Build history of the part. All positions in model axes, mm. Face numbers are marked on the shaded views. Round coordinates to 2 decimals unless told otherwise and drop trailing zeros. Loops run counter-clockwise (first coordinate to the right, second up) from the corner with the lowest first, then second, coordinate; pieces in that order, holes last.
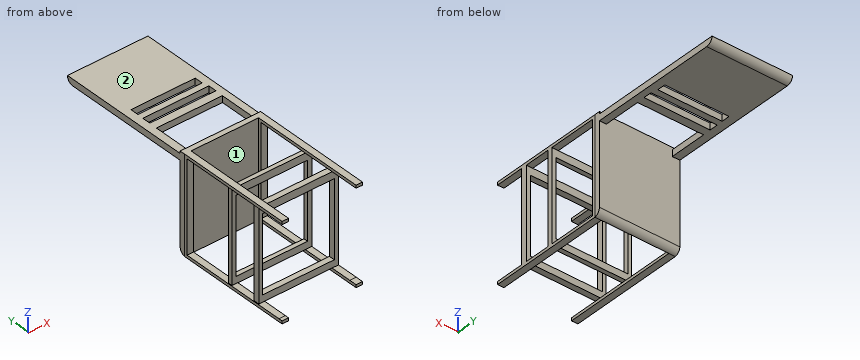
from build123d import *

# Parameters (mm, degrees)
SKETCH1_W                = 25.4
SKETCH1_H                = 381
BOSS_EXTRUDE1_DEPTH      = 457.2
BOSS_EXTRUDE1_2_DEPTH    = 457.2
SKETCH5_W                = 358.329211732
SKETCH5_H                = 431.015208417
CUT_EXTRUDE1_DEPTH       = 457.2
BOSS_EXTRUDE7_DEPTH      = 35.814
BOSS_EXTRUDE7_DEPTH_BACK = 281.94
SKETCH13_W               = 381.141342185
SKETCH13_H               = 21.019014934
SKETCH14_W               = 317.754
SKETCH14_H               = 526.086170676
BOSS_EXTRUDE8_DEPTH      = 25.4
SKETCH17_W               = 260.552131225
SKETCH17_H               = 146.876016362
SKETCH17_H_2             = 29.104227424
CUT_EXTRUDE3_DEPTH       = 25.4
BOSS_EXTRUDE9_DEPTH      = 25.4
SKETCH19_W               = 260.972204044
SKETCH19_H               = 32.78881538
SKETCH19_W_2             = 254
CUT_EXTRUDE6_DEPTH       = 35.56
FILLET1_R                = 25.4
FILLET2_R                = 25.4
SKETCH20_W               = 358.469269341
SKETCH20_H               = 15.323983409
CUT_EXTRUDE7_DEPTH       = 288.544
SKETCH21_W               = 358.469269341
SKETCH21_H               = 29.641446852
CUT_EXTRUDE8_DEPTH       = 80.772
BOSS_EXTRUDE10_START     = -279.146
SKETCH22_W               = 358.329211732
SKETCH22_H               = 17.235921955
SKETCH22_H_2             = 22.86
BOSS_EXTRUDE10_DEPTH     = 314.887549
CUT_EXTRUDE9_DEPTH       = 378.46
CUT_EXTRUDE9_DEPTH_BACK  = 279.146
SKETCH23_W               = 283.569919334
SKETCH23_H               = 301.695006961
SKETCH24_W               = 411.753611465
SKETCH24_H               = 408.769889643
CUT_EXTRUDE11_DEPTH      = 75.946
FILLET3_R                = 25.4


# Some blends are built 0.0001 mm under size
with BuildPart() as part:
    # Sketch1 → Boss-Extrude1 (new body)
    with BuildSketch(Plane(origin=(0, 0, 0), x_dir=(1, 0, 0), z_dir=(0, 1, 0))):
        with Locations((-269.080936413, 156.123579529)):
            Rectangle(SKETCH1_W, SKETCH1_H)
    extrude(amount=BOSS_EXTRUDE1_DEPTH)


with BuildPart() as body_2:
    # Sketch1 → Boss-Extrude1 2 (new body)
    with BuildSketch(Plane(origin=(0, 0, 0), x_dir=(1, 0, 0), z_dir=(0, 1, 0))):
        with Locations((23.041549082, 156.123579529)):
            Rectangle(SKETCH1_W, SKETCH1_H)
    extrude(amount=BOSS_EXTRUDE1_2_DEPTH)


with BuildPart() as cut_extrude1_tool:
    # Sketch5 → Cut-Extrude1 (new body)
    with BuildSketch(Plane(origin=(35.741549082, 0, 0), x_dir=(0, 0, -1), z_dir=(1, 0, 0))):
        with Locations((156.123579529, 230.831587618)):
            Rectangle(SKETCH5_W, SKETCH5_H)
    extrude(amount=-CUT_EXTRUDE1_DEPTH)


with BuildPart() as part_1:
    add(part.part)

    # Cut-Extrude1: cut by cut_extrude1_tool
    add(cut_extrude1_tool.part, mode=Mode.SUBTRACT)



with BuildPart() as body_2_1:
    add(body_2.part)

    # Cut-Extrude1: cut by cut_extrude1_tool
    add(cut_extrude1_tool.part, mode=Mode.SUBTRACT)


with BuildPart() as part_2:
    add(part_1.part)

    add(body_2_1.part)  # Boss-Extrude7 merges body 2
    # Sketch13 → Boss-Extrude7 (add, two sides: drawn at the far end of the back side and taken through both)
    with BuildSketch(Plane(origin=(0, 0, 0), x_dir=(0, 0, -1), z_dir=(1, 0, 0)).offset(-BOSS_EXTRUDE7_DEPTH_BACK)):
        with Locations((156.194250622, 467.709507467)):
            Rectangle(SKETCH13_W, SKETCH13_H)
    extrude(amount=BOSS_EXTRUDE7_DEPTH + BOSS_EXTRUDE7_DEPTH_BACK)

    # Sketch14 → Boss-Extrude8 (add)
    with BuildSketch(Plane.XY):
        with Locations((-123.063, 730.752592805)):
            Rectangle(SKETCH14_W, SKETCH14_H)
    extrude(amount=BOSS_EXTRUDE8_DEPTH)

    # Sketch17 → Cut-Extrude3 (cut)
    with BuildSketch(Plane.XY.offset(25.4)):
        with Locations((-121.677084409, 551.657023115)):
            Rectangle(SKETCH17_W, SKETCH17_H)
        with Locations((-121.677084409, 663.207710066)):
            Rectangle(SKETCH17_W, SKETCH17_H_2)
        with Locations((-121.677084409, 710.328840181)):
            Rectangle(SKETCH17_W, SKETCH17_H_2)
    extrude(amount=-CUT_EXTRUDE3_DEPTH, mode=Mode.SUBTRACT)

    # Sketch18 → Boss-Extrude9 (add)
    with BuildSketch(Plane.XY):
        Polygon((-281.94, 993.795678143), (-281.94, 1247.795678143), (35.814, 1247.795678143), (35.814, 993.795678143), (35.814, 478.219014934), (8.598981204, 478.219014934), (8.598981204, 625.095031296), (-251.953150021, 625.095031296), (-251.953150021, 478.219014934), (-281.94, 478.219014934), align=None)
    extrude(amount=BOSS_EXTRUDE9_DEPTH)

    # Sketch19 → Cut-Extrude6 (cut)
    with BuildSketch(Plane.XY):
        with Locations((-120.300778352, 673.69810694)):
            Rectangle(SKETCH19_W, SKETCH19_H)
        with Locations((-122.448561379, 731.24582373)):
            Rectangle(SKETCH19_W_2, SKETCH19_H)
    extrude(amount=CUT_EXTRUDE6_DEPTH, mode=Mode.SUBTRACT)

    # Fillet1
    fillet1_edges = [part_2.edges().sort_by_distance(p)[0] for p in [
        (-123.063, 1247.795678143, 0),
    ]]
    fillet(fillet1_edges, radius=FILLET1_R - 0.0001)  # a hair under: the kernel refuses the full size

    # Fillet2
    # the kernel refuses this fillet: 25.4 mm, written as the material it takes off along each edge
    with BuildSketch(Plane(origin=(-344.488329806, 478.219014934, -346.764921714), x_dir=(0, 0, 1), z_dir=(1, 0, 0))) as fillet2_piece_1:
        with BuildLine():
            CenterArc((25.019331923, 25.4), FILLET2_R, 189.932027033, 80.067972967)
            Line((0, 21.019014934), (-0.500386638, 20.931395233))
            ThreePointArc((-0.500386638, 20.931395233), (-0.508, 10.509507467), (-0.508, 0))
            Line((-0.508, 0), (0, -0.508))
            Line((0, -0.508), (25.019331923, -0.508))
            Line((25.019331923, -0.508), (25.019331923, 0))
        make_face()
    extrude(amount=442.850659613, mode=Mode.SUBTRACT)

    # Sketch20 → Cut-Extrude7 (cut)
    with BuildSketch(Plane(origin=(0, 0, 0), x_dir=(0, 0, -1), z_dir=(1, 0, 0))):
        with Locations((156.193608334, 7.661991705)):
            Rectangle(SKETCH20_W, SKETCH20_H)
    extrude(amount=-CUT_EXTRUDE7_DEPTH, mode=Mode.SUBTRACT)

    # Sketch21 → Cut-Extrude8 (cut)
    with BuildSketch(Plane(origin=(0, 0, 0), x_dir=(0, 0, -1), z_dir=(1, 0, 0))):
        with Locations((156.193608334, 14.820723426)):
            Rectangle(SKETCH21_W, SKETCH21_H)
    extrude(amount=CUT_EXTRUDE8_DEPTH, mode=Mode.SUBTRACT)

    # Sketch22 → Boss-Extrude10 (add)
    with BuildSketch(Plane(origin=(0, 0, 0), x_dir=(0, 0, -1), z_dir=(1, 0, 0)).offset(BOSS_EXTRUDE10_START)):
        with Locations((156.123579529, 246.608280317)):
            Rectangle(SKETCH22_W, SKETCH22_H)
        with Locations((156.123579529, 124.076015291)):
            Rectangle(SKETCH22_W, SKETCH22_H_2)
    extrude(amount=BOSS_EXTRUDE10_DEPTH)

    # Sketch23 → Cut-Extrude9 (cut, two sides: drawn at the far end of the back side and taken through both)
    with BuildSketch(Plane(origin=(0, 0, 0), x_dir=(1, 0, 0), z_dir=(0, 1, 0)).offset(-CUT_EXTRUDE9_DEPTH_BACK)):
        with Locations((-122.770659877, 157.655951237)):
            Rectangle(SKETCH23_W, SKETCH23_H)
    extrude(amount=CUT_EXTRUDE9_DEPTH + CUT_EXTRUDE9_DEPTH_BACK, mode=Mode.SUBTRACT)

    # Sketch24 → Cut-Extrude11 (cut)
    with BuildSketch(Plane.XY.offset(25.4)):
        with Locations((-113.714072953, 1211.167180329)):
            Rectangle(SKETCH24_W, SKETCH24_H)
    extrude(amount=-CUT_EXTRUDE11_DEPTH, mode=Mode.SUBTRACT)

    # Fillet3
    fillet3_edges = [part_2.edges().sort_by_distance(p)[0] for p in [
        (-123.063, 1006.782235507, 0),
    ]]
    fillet(fillet3_edges, radius=FILLET3_R - 0.0001)  # a hair under: the kernel refuses the full size


solid = part_2.part
(1) Pin check, flat tips, straight feed: P1, Ø1.5, axis at x = -195, z = -182.5, coming from the +Y side; P2, Ø20.5, axis at x = 25, y = 306.5, coming from the -Z side; P3, Ø25, axis at y = 124, z = -71, coming from the -X side. Stop position of each tip, or through.
Responses:
P1: stops at y = 478.22
P2: stops at z = -346.62
P3: stops at x = -279.15
(2) Slice it at C-C on y = 610. List the corners of the cut face in (x, z).
Responses:
outline: (-281.94, 0) - (-251.95, 0) - (-251.95, 25.4) - (-281.94, 25.4) - close; (8.6, 0) - (35.81, 0) - (35.81, 25.4) - (8.6, 25.4) - close
(3) Slice it at A-A on x = -175. Count the separate pieces of the cut face and the enclosed holes in it, plus the area to 3 significant figures.
Responses:
separate pieces: 8
enclosed holes: 0
area: 18,000 mm2
(4) Pull direction X, two halves, no side cores. Call the marked faces 1 and 2: +X half, -X half, draft (parallel to the pull), parting line (faces both ways), or undercut.
Responses:
face 1: undercut
face 2: draft
(5) Slice it at D-D on y = 881. List the corners of the cut face in (x, z), plus the area to 3 significant figures.
Responses:
outline: (-281.94, 0) - (35.81, 0) - (35.81, 25.4) - (-281.94, 25.4) - close
area: 8,070 mm2
(6) Probe line 1 (Y direction, x = -51.5, z = -318); line 2 (X direction, y = 114, z = -106); line 3 (Z direction, x = -238, y = 657). List the from-to ranges inside material, lowest first.
Responses:
line 1: y = 112.65 to 135.51, 237.99 to 255.23, 457.2 to 478.22
line 2: x = -279.15 to -264.56, 19.01 to 35.74
line 3: z = 0 to 25.4
(7) Slice it at B-B on z = -171. List the corners of the cut face in (x, y), plus the area to 3 significant figures.
Responses:
outline: (-281.94, 457.2) - (-281.78, 457.2) - (-281.78, 446.34) - (-256.38, 446.34) - (-256.38, 457.2) - (10.34, 457.2) - (10.34, 446.34) - (35.74, 446.34) - (35.74, 457.2) - (35.81, 457.2) - (35.81, 478.22) - (-281.94, 478.22) - close; (-279.15, 112.65) - (-264.56, 112.65) - (-264.56, 135.51) - (-279.15, 135.51) - close; (-279.15, 237.99) - (-264.56, 237.99) - (-264.56, 255.23) - (-279.15, 255.23) - close; (19.01, 112.65) - (35.74, 112.65) - (35.74, 135.51) - (19.01, 135.51) - close; (19.01, 237.99) - (35.74, 237.99) - (35.74, 255.23) - (19.01, 255.23) - close
area: 8,490 mm2
